Geometry check sheet. Reference: the model listing, model coordinates, mm. A direction names the side the tool comes from. Round coordinates to 2 decimals unless told otherwise and drop trailing zeros. Loops run counter-clockwise (first coordinate to the right, second up) from the corner with the lowest first, then second, coordinate; pieces in that order, holes last. Notation, with made-up numbers: M 56.25,-36 L 84.25,-36 A21 cw 84.25,-16 Z; hole C 20.25,73.25 d9. An arc over 180 degrees is marked long. Write item = value, one per line.
Autodesk Inventor part; units mm, degrees
ref_plane "YZ Plane" through (0, 0, 0) normal (1, 0, 0) x (0, 1, 0)
ref_plane "XZ Plane" through (0, 0, 0) normal (0, 1, 0) x (-1, 0, 0)
ref_plane "XY Plane" through (0, 0, 0) normal (0, 0, 1) x (1, 0, 0)
sketch "スケッチ1" plane through (0, 0, 0) normal (0, 0, 1) x (1, 0, 0)
  line L0 (-12.5, 25) -> (12.5, 25)
  line L1 (12.5, 25) -> (12.5, 0)
  line L2 (12.5, 0) -> (-12.5, 0)
  line L3 (-12.5, 0) -> (-12.5, 25)
  line L4 (-10.5, 25) -> (10.5, 25)
  line L5 (10.5, 25) -> (10.5, 2)
  line L6 (10.5, 2) -> (-10.5, 2)
  line L7 (-10.5, 2) -> (-10.5, 25)
  point P0 (0, 0)
  dimension "d0" = 25
  dimension "d1" = 25
  dimension "d2" = 0
  dimension "d3" = 12.5
  dimension "d4" = 2
  dimension "d5" = 2
  dimension "d6" = 2
extrude "押し出し1" add sketch "スケッチ1" along normal blind 36 contours L0 L7 L6 L5 L1 L2 L3
sketch "スケッチ2" plane through (12.5, 0, 0) normal (1, 0, 0) x (0, 0, -1)
  line L0 (-36, 25) -> (-36, 0)
  line L1 (0, 25) -> (-36, 25)
  point P0 (-28, 17)
  point P1 (-8, 17)
  dimension "d9" = 20
  dimension "d10" = 8
  dimension "d11" = 8
  dimension "d12" = 8
hole "Hole1" at (12.5, 17, 28) at (12.5, 17, 8) direction (-1, 0, 0) diameter 6 end through all
fillet "フィレット1" radius 8 4 edges at (11.5, 25, 36) (-11.5, 25, 36) (-11.5, 25, 0) (11.5, 25, 0)
sketch "スケッチ3" plane through (-10.5, 2, 36) normal (0, 1, 0) x (1, 0, 0)
  line L0 (21, 0) -> (0, 0)
  line L1 (21, 36) -> (21, 0)
  line L2 (0, 36) -> (21, 36)
  line L3 (0, 36) -> (0, 0)
  point P0 (10.5, 36)
  point P1 (4, 30)
  point P2 (17, 30)
  point P3 (17, 6)
  point P4 (4, 6)
  dimension "d21" = 6
  dimension "d22" = 4
  dimension "d23" = 6
  dimension "d24" = 4
  dimension "d25" = 4
  dimension "d26" = 6
  dimension "d27" = 6
  dimension "d28" = 4
hole "Hole2" at (-6.5, 2, 6) at (6.5, 2, 6) at (6.5, 2, 30) at (-6.5, 2, 30) direction (0, -1, 0) diameter 3.2 end through all
sketch "スケッチ4" plane through (-12.5, 0, 0) normal (0, -1, 0) x (1, 0, 0)
  line L0 (0, 0) -> (0, 36)
  line L1 (25, 0) -> (25, 36)
  line L2 (25, 18) -> (0, 18)
  line L3 (0, 24.05) -> (25, 24.05)
  line L4 (25, 24.05) -> (25, 11.95)
  line L5 (25, 11.95) -> (0, 11.95)
  line L6 (0, 11.95) -> (0, 24.05)
  point P0 (12.5, 0)
  dimension "d36" = 12.1
  dimension "d37" = 12.1
extrude "押し出し2" cut sketch "スケッチ4" against normal blind 2.1
equation "\"d1\" = d0"
equation "\"d5\" = d4"
equation "\"d6\" = d4"
equation "\"d37\" = d36"
properties part number "JointC3_2nd" material "アルミニウム 6061"
(1) Sectioned sample at B-B on x = -1. Record the cut outline in (y, z).
Result set:
outline = M 0,0 L 2,0 L 2,11.95 L 0,11.95 Z; M 0,24.05 L 2,24.05 L 2,36 L 0,36 Z
(2) Tool access check on faces 1 (the cylindrical face through (7.47, 0.99, 28.73)), 2 (the flat face through (0, 2, 30)), 3 (the flat face through (0, 1, 24.05)). Record the directions out of +Z, -Z, +X, -X, +Y, -Y that give a thin tool (end or side, any length) a straight path to the whole face; none if there is none.
Result set:
face_1 = +Y, -Y
face_2 = +Z, -Z, +Y
face_3 = +X, -X, -Y
(3) Sectioned sample at D-D on y = 16.5. Record the cut outline in (x, z), then the cut area to 3 significant figures.
Result set:
outline = M -12.5,0 L -10.5,0 L -10.5,5.04 L -12.5,5.04 Z; M -12.5,10.96 L -10.5,10.96 L -10.5,25.04 L -12.5,25.04 Z; M -12.5,30.96 L -10.5,30.96 L -10.5,36 L -12.5,36 Z; M 10.5,0 L 12.5,0 L 12.5,5.04 L 10.5,5.04 Z; M 10.5,10.96 L 12.5,10.96 L 12.5,25.04 L 10.5,25.04 Z; M 10.5,30.96 L 12.5,30.96 L 12.5,36 L 10.5,36 Z
area = 96.7 mm2
(4) Depth check by flat-ended pin: pin 1 Ø2 at (x, z) = (11.5, 17) entering from -Y; pin 2 Ø9.5 at (y, z) = (17, 8) entering from +X; pin 3 Ø3.5 at (x, z) = (4.5, 5.5) entering from +Y. Enter the tip coordinate at first touch or a pass-through.
Result set:
pin_1 = 2.1
pin_2 = 12.5
pin_3 = 2
(5) Sectioned sample at C-C on x = 6.5. Record the cut outline in (y, z), then the cut area to 3 significant figures.
Result set:
outline = M 0,0 L 2,0 L 2,4.4 L 0,4.4 Z; M 0,7.6 L 2,7.6 L 2,11.95 L 0,11.95 Z; M 0,24.05 L 2,24.05 L 2,28.4 L 0,28.4 Z; M 0,31.6 L 2,31.6 L 2,36 L 0,36 Z
area = 35.0 mm2
(6) Material ranges on line 1 along Z through (x, y) = (11.35, 17); line 2 along X through (y, z) = (1.55, 30); line 3 along X through (y, z) = (6.25, 21.5), recorded low to high. Write a range as from..to.
Result set:
line_1 = 0..5, 11..25, 31..36
line_2 = -12.5..-8.1, -4.9..4.9, 8.1..12.5
line_3 = -12.5..-10.5, 10.5..12.5
(7) Release check for a two-part mould opening along X. For faces 4 (the flat face through (0.9, 1.6, 36)), 5 (the flat face through (-12.5, 12, 18)), 6 (the flat face through (-10.5, 13, 18)) record: released by +X, released by -X, zero draft, split by the parting line, or undercut.
Result set:
face_4 = zero draft
face_5 = released by -X
face_6 = undercut
(8) Sectioned sample at A-A on z = 23. Record the cut outline in (x, y).
Result set:
outline = M -12.5,2.1 L -10.5,2.1 L -10.5,25 L -12.5,25 Z; M 10.5,2.1 L 12.5,2.1 L 12.5,25 L 10.5,25 Z
